Check sheet for the modelled part. Datum: model origin and axes. Units: mm. A direction names the side the tool comes from. Coordinates: 2 decimals unless noted, no trailing zeros. Order: outer loops, then holes, each group sorted by start corner. A loop starts at its lowest first (then second) coordinate and runs counter-clockwise, first axis right, second up.
from build123d import *

# Parameters (mm, degrees)
SKETCH1_W                       = 80
SKETCH1_H                       = 65
BOSS_EXTRUDE1_DEPTH             = 20
SKETCH2_W                       = 70
SKETCH2_H                       = 61
CUT_EXTRUDE1_DEPTH              = 15
CUT_EXTRUDE7_REACH              = 80.899
SKETCH9_W                       = 70
SKETCH9_H                       = 15
BOSS_EXTRUDE2_DEPTH             = 10.125
SKETCH3_3_W                     = 3
SKETCH3_3_H                     = 6.1
BOSS_EXTRUDE3_DEPTH             = 2
TAP_DRILL_FOR_M2X0_4_TAP1_D     = 1.6
TAP_DRILL_FOR_M2X0_4_TAP1_DEPTH = 5
TAP_DRILL_FOR_M2X0_4_TAP1_TIP   = 0.480688495
CUT_EXTRUDE2_REACH              = 90.635
SKETCH7_R                       = 8.2
SKETCH7_3_R                     = 9.5
CUT_EXTRUDE3_DEPTH              = 1
SKETCH7_4_R                     = 8.2
CUT_EXTRUDE4_DEPTH              = 89.635489506
SKETCH7_5_R                     = 9.5
SKETCH7_5_R_2                   = 8.2
CUT_EXTRUDE5_DEPTH              = 1
CUT_EXTRUDE6_DEPTH              = 56.283360969
CUT_EXTRUDE6_DEPTH_BACK         = 56.283360969
SKETCH8_W                       = 15
SKETCH8_H                       = 57.5
TAP_DRILL_FOR_M2X0_4_TAP2_D     = 1.8
TAP_DRILL_FOR_M2X0_4_TAP2_DEPTH = 10
TAP_DRILL_FOR_M2X0_4_TAP2_TIP   = 0.540774557


with BuildPart() as part:
    # Sketch1 → Boss-Extrude1 (new body)
    with BuildSketch(Plane.XY):
        Rectangle(SKETCH1_W, SKETCH1_H)
    extrude(amount=BOSS_EXTRUDE1_DEPTH)

    # Sketch2 → Cut-Extrude1 (cut)
    with BuildSketch(Plane.XY.offset(20)):
        Rectangle(SKETCH2_W, SKETCH2_H)
    extrude(amount=-CUT_EXTRUDE1_DEPTH, mode=Mode.SUBTRACT)

    # Sketch9 → Cut-Extrude7 (cut, up to next)
    with BuildSketch(Plane(origin=(0, 32.5, 0), x_dir=(1, 0, 0), z_dir=(0, 1, 0)), mode=Mode.PRIVATE) as cut_extrude7_sk1:
        with Locations((0, -12.5)):
            Rectangle(SKETCH9_W, SKETCH9_H)
    cut_extrude7_tool1 = extrude(cut_extrude7_sk1.sketch, amount=-CUT_EXTRUDE7_REACH, mode=Mode.PRIVATE) & part.part
    add(cut_extrude7_tool1.solids().sort_by_distance((0, 32.5, 12.5))[0], mode=Mode.SUBTRACT)

    # Sketch3 → Boss-Extrude2 (add)
    with BuildSketch(Plane.XY.offset(5)):
        Polygon((12.923634865, 20.4), (-14.276365135, 20.4), (-14.276365135, 17.4), (9.923634865, 17.4), (12.923634865, 17.4), align=None)
        Polygon((12.923634865, 5.2), (9.923634865, 5.2), (-14.276365135, 5.2), (-14.276365135, 2.2), (12.923634865, 2.2), align=None)
    extrude(amount=BOSS_EXTRUDE2_DEPTH)

    # Sketch3<3> → Boss-Extrude3 (add)
    with BuildSketch(Plane.XY.offset(5)):
        with Locations((11.423634865, 14.35)):
            Rectangle(SKETCH3_3_W, SKETCH3_3_H)
        with Locations((11.423634865, 8.25)):
            Rectangle(SKETCH3_3_W, SKETCH3_3_H)
    extrude(amount=BOSS_EXTRUDE3_DEPTH)

    # Tap Drill for M2x0.4 Tap1
    with Locations(Plane.XY.offset(15.125)):
        with Locations((-9.276365135, 18.9), (0.723634865, 18.9), (0.723634865, 3.7), (-9.276365135, 3.7)):
            Hole(TAP_DRILL_FOR_M2X0_4_TAP1_D / 2, depth=TAP_DRILL_FOR_M2X0_4_TAP1_DEPTH)
            with Locations((0, 0, -(TAP_DRILL_FOR_M2X0_4_TAP1_DEPTH + TAP_DRILL_FOR_M2X0_4_TAP1_TIP / 2))):  # 118° drill point
                Cone(0, TAP_DRILL_FOR_M2X0_4_TAP1_D / 2, TAP_DRILL_FOR_M2X0_4_TAP1_TIP, mode=Mode.SUBTRACT)

    # Cut-Extrude2: up to this face of the body (flat: up to its plane)
    cut_extrude2_end = Plane(part.part.faces().sort_by_distance((-14.276365135, 18.9, 10.0625))[0])
    # Sketch7 → Cut-Extrude2 (cut, up to the picked face)
    with BuildSketch(Plane.ZY.offset(40), mode=Mode.PRIVATE) as cut_extrude2_sk1:
        with Locations((10, 11.3)):
            Circle(SKETCH7_R)
    cut_extrude2_tool1 = split(extrude(cut_extrude2_sk1.sketch, amount=-CUT_EXTRUDE2_REACH, mode=Mode.PRIVATE), bisect_by=cut_extrude2_end, keep=Keep.BOTH, mode=Mode.PRIVATE)
    add(cut_extrude2_tool1.solids().sort_by(Axis((-40, 11.3, 10), (1, 0, 0)))[0], mode=Mode.SUBTRACT)

    # Sketch7<3> → Cut-Extrude3 (cut)
    with BuildSketch(Plane.ZY.offset(40)):
        with Locations((10, 11.3)):
            Circle(SKETCH7_3_R)
    extrude(amount=-CUT_EXTRUDE3_DEPTH, mode=Mode.SUBTRACT)

    # Sketch7<4> → Cut-Extrude4 (cut, through all)
    with BuildSketch(Plane.ZY.offset(40)):
        with Locations((10, -20)):
            Circle(SKETCH7_4_R)
    extrude(amount=-CUT_EXTRUDE4_DEPTH, mode=Mode.SUBTRACT)

    # Sketch7<5> → Cut-Extrude5 (cut)
    with BuildSketch(Plane.ZY.offset(40)):
        with Locations((10, -20)):
            Circle(SKETCH7_5_R)
        with Locations((10, -20)):
            Circle(SKETCH7_5_R_2, mode=Mode.SUBTRACT)
    cut_extrude5 = extrude(amount=-CUT_EXTRUDE5_DEPTH, mode=Mode.SUBTRACT)

    # Mirror1: Cut-Extrude5 across plane
    add(cut_extrude5.mirror(Plane(origin=(0, 0, 0), x_dir=(0, 0, 1), z_dir=(1, 0, 0))), mode=Mode.SUBTRACT)

    # Sketch8 → Cut-Extrude6 (cut, two sides: drawn at the far end of the back side and taken through both)
    with BuildSketch(Plane(origin=(0, 0, 0), x_dir=(-1, 0, 0), z_dir=(0, 0, -1)).offset(-CUT_EXTRUDE6_DEPTH_BACK)):
        with Locations((24.276365135, -20)):
            Rectangle(SKETCH8_W, SKETCH8_H)
        with Locations((-24.276365135, -20)):
            Rectangle(SKETCH8_W, SKETCH8_H)
    extrude(amount=CUT_EXTRUDE6_DEPTH + CUT_EXTRUDE6_DEPTH_BACK, mode=Mode.SUBTRACT)

    # Tap Drill for M2x0.4 Tap2
    with Locations(Plane(origin=(0, 32.5, 0), x_dir=(1, 0, 0), z_dir=(0, 1, 0))):
        with Locations((-37.5, -17.5), (-37.5, -2.5), (37.5, -2.5), (37.5, -17.5)):
            Hole(TAP_DRILL_FOR_M2X0_4_TAP2_D / 2, depth=TAP_DRILL_FOR_M2X0_4_TAP2_DEPTH)
            with Locations((0, 0, -(TAP_DRILL_FOR_M2X0_4_TAP2_DEPTH + TAP_DRILL_FOR_M2X0_4_TAP2_TIP / 2))):  # 118° drill point
                Cone(0, TAP_DRILL_FOR_M2X0_4_TAP2_D / 2, TAP_DRILL_FOR_M2X0_4_TAP2_TIP, mode=Mode.SUBTRACT)


solid = part.part
(1) Go/stop test with flat-tipped pins: P1, Ø6, axis at x = -3.5, y = -12.5, coming from the +Z side; P2, Ø4.5, axis at x = 7, z = 9, coming from the +Y side; P3, Ø10, axis at x = 4.5, z = 7, coming from the +Y side; P4, Ø3, axis at x = -26.5, z = 7.5, coming from the -Y side. Record where each tip stops, or that it passes through.
Filled in:
P1: stops at z = 5
P2: stops at y = 20.4
P3: stops at y = 32.5
P4: passes through
(2) Cross-section at A-A (y = -6.5). Enter the section's corners in (x, z).
Filled in:
outline: (-40, 0) - (-31.78, 0) - (-31.78, 5) - (-35, 5) - (-35, 20) - (-40, 20) - close; (-16.78, 0) - (16.78, 0) - (16.78, 5) - (-16.78, 5) - close; (31.78, 0) - (40, 0) - (40, 20) - (35, 20) - (35, 5) - (31.78, 5) - close
(3) Cross-section at C-C (x = 23). Enter the section's corners in (y, z), and give its area (3 significant figures).
Filled in:
outline: (8.75, 0) - (32.5, 0) - (32.5, 5) - (8.75, 5) - close
area: 119 mm2
(4) Release check for a two-part mould opening along Y. For faces 5 (the conical face through (37.344, 22.053, 17.493)), 6 (the flat face through (35, 8, 13)), 7 (the cylindrical face through (-9.1, 18.12, 12.59)) record: +Y half, -Y half, draft (parallel to the pull), parting line (faces both ways), or undercut.
Filled in:
face 5: +Y half
face 6: draft
face 7: undercut
(5) Cross-section at B-B (x = -4). Enter the section's corners in (y, z) (3 decimals).
Filled in:
outline: (-32.5, 0) - (32.5, 0) - (32.5, 5) - (20.4, 5) - (20.4, 15.125) - (17.4, 15.125) - (17.4, 5) - (5.2, 5) - (5.2, 15.125) - (2.2, 15.125) - (2.2, 5) - (-13.501, 5) arc R8.2 cw to (-26.499, 5) - (-30.5, 5) - (-30.5, 20) - (-32.5, 20) - close
(6) Thickness scan on probe 1 along Y at (x, z) = (4, 8.25); probe 2 along X at (y, z) = (3.7, 13.9); probe 3 along Z at (x, y) = (-37.5, 27.5). Record the ranges inside material, lowest first.
Filled in:
probe 1: y = -32.5 to -30.5, 2.2 to 5.2, 17.4 to 20.4
probe 2: x = -39 to -35, -14.28 to -10.08, -8.48 to -0.08, 1.52 to 12.92, 35 to 40
probe 3: z = 0 to 1.6, 3.4 to 16.6, 18.4 to 20
(7) Tool access check on faces 1 (the flat face through (11, 11, 7)), 2 (the flat face through (-1, 4, 15.125)), 3 (the cylindrical face through (-29.558, 11.661, 1.808)), 4 (the flat face through (24, 8.75, 3)). Record the directions out of +Z, -Z, +X, -X, +Y, -Y that give a thin tool (end or side, any length) a straight path to the whole face; none if there is none.
Filled in:
face 1: +Z, -X
face 2: +Z, +Y
face 3: -X
face 4: +Z, -Z, -Y
